Part model, mm, in its own coordinate system. A direction names the side the tool comes from. Round coordinates to 2 decimals unless told otherwise and drop trailing zeros. Order: outer loops, then holes, each group sorted by start corner. A loop starts at its lowest first (then second) coordinate and runs counter-clockwise, first axis right, second up. Notation, with made-up numbers: M -21,86.25 L 0,86.25 A15 cw 0,114.25 Z; hole C 51,45.5 d6. An arc over 180 degrees is marked long. One line per question, with ' | ' between items.
from build123d import *

# Parameters (mm, degrees)
BASE_FLANGE1_DEPTH      = 12.5
CUT_EXTRUDE2_DEPTH      = 64.602279833
CUT_EXTRUDE2_DEPTH_BACK = 64.602279833
SKETCH7_R               = 1.3
SKETCH16_R              = 5
CUT_EXTRUDE5_DEPTH      = 10
SKETCH17_R              = 1.3
CUT_EXTRUDE6_DEPTH      = 10
FILLET3_R               = 2
SKETCH18_W              = 7
SKETCH18_H              = 42.8
CUT_EXTRUDE7_DEPTH      = 71.087445381
FILLET4_R               = 2


# Sheet-metal steps are written as plain solids
with BuildPart() as part:
    # Sketch1 → Base-Flange1 (new, symmetric)
    with BuildSketch(Plane.XY):
        with BuildLine():
            Line((-15, 60), (-15, 3.33))
            ThreePointArc((-15, 3.33), (-14.024665581, 0.975334419), (-11.67, 0))
            Line((-11.67, 0), (11.67, 0))
            ThreePointArc((11.67, 0), (14.024665581, 0.975334419), (15, 3.33))
            Line((15, 3.33), (15, 60))
            Line((15, 60), (17, 60))
            Line((17, 60), (17, 3.33))
            ThreePointArc((17, 3.33), (15.438879144, -0.438879144), (11.67, -2))
            Line((11.67, -2), (-11.67, -2))
            ThreePointArc((-11.67, -2), (-15.438879144, -0.438879144), (-17, 3.33))
            Line((-17, 3.33), (-17, 60))
            Line((-17, 60), (-15, 60))
        make_face()
    extrude(amount=BASE_FLANGE1_DEPTH, both=True)

    # Sketch7 → Cut-Extrude2 (cut, two sides: drawn at the far end of the back side and taken through both)
    with BuildSketch(Plane(origin=(0, 0, 0), x_dir=(0, 0, -1), z_dir=(1, 0, 0)).offset(-CUT_EXTRUDE2_DEPTH_BACK)):
        with Locations((-8.5, 57.4)):
            Circle(SKETCH7_R)
        with Locations((8.5, 57.4)):
            Circle(SKETCH7_R)
    extrude(amount=CUT_EXTRUDE2_DEPTH + CUT_EXTRUDE2_DEPTH_BACK, mode=Mode.SUBTRACT)

    # Sketch16 → Cut-Extrude5 (cut)
    with BuildSketch(Plane.XZ.offset(2)):
        with Locations(Location((0, 0, 0), (0, 0, 270))):
            Circle(SKETCH16_R)
    extrude(amount=-CUT_EXTRUDE5_DEPTH, mode=Mode.SUBTRACT)

    # Sketch17 → Cut-Extrude6 (cut)
    with BuildSketch(Plane(origin=(0, 0, 0), x_dir=(1, 0, 0), z_dir=(0, 1, 0))):
        with Locations(Location((-9, 10, 0), (0, 0, 270))):
            Circle(SKETCH17_R)
        with Locations(Location((9, 10, 0), (0, 0, 270))):
            Circle(SKETCH17_R)
        with Locations(Location((9, -10, 0), (0, 0, 270))):
            Circle(SKETCH17_R)
        with Locations(Location((-9, -10, 0), (0, 0, 270))):
            Circle(SKETCH17_R)
    extrude(amount=-CUT_EXTRUDE6_DEPTH, mode=Mode.SUBTRACT)

    # Fillet3
    fillet3_edges = [part.edges().sort_by_distance(p)[0] for p in [
        (-16, 60, -12.5),
        (16, 60, -12.5),
        (-16, 60, 12.5),
        (16, 60, 12.5),
    ]]
    fillet(fillet3_edges, radius=FILLET3_R)

    # Sketch18 → Cut-Extrude7 (cut, through all)
    with BuildSketch(Plane.ZY.offset(17)):
        with Locations((0, 30)):
            Rectangle(SKETCH18_W, SKETCH18_H)
    extrude(amount=-CUT_EXTRUDE7_DEPTH, mode=Mode.SUBTRACT)

    # Fillet4
    fillet4_edges = [part.edges().sort_by_distance(p)[0] for p in [
        (16, 51.4, 3.5),
        (16, 8.6, 3.5),
        (16, 8.6, -3.5),
        (16, 51.4, -3.5),
        (-16, 51.4, 3.5),
        (-16, 8.6, 3.5),
        (-16, 8.6, -3.5),
        (-16, 51.4, -3.5),
    ]]
    fillet(fillet4_edges, radius=FILLET4_R)


solid = part.part
1) Probe line 1 (X direction, y = 15, z = 10); line 2 (Z direction, x = -15.6, y = 57.4); line 3 (X direction, y = -0.6, z = 10). List the from-to ranges inside material, lowest first. Write a range as [from, to].
The answers:
line 1: x = [-17, -15], [15, 17] | line 2: z = [-12.5, -9.8], [-7.2, 7.2], [9.8, 12.5] | line 3: x = [-15.27, -10.3], [-7.7, 7.7], [10.3, 15.27]
2) Two-plate mould, pull along Y, no slides. Class faces 1 (the face through (16, 8.6, 0)), 2 (the face through (9.39, -0.99, -8.76)), 3 (the face through (-15.99, 50.8, 2.93)), 4 (the face through (-15.4, -0.48, 0.18)): released by +Y, released by -Y, zero draft, split by the parting line, or undercut.
The answers:
face 1: undercut | face 2: zero draft | face 3: undercut | face 4: released by -Y
3) Drop flat-ended pins along their axis: pin 1 (0.6 mm diameter, centred on x = 16, z = 0.5, fed in from -Y); pin 2 (8 mm diameter, centred on x = 9, z = -1, fed in from +Y); pin 3 (3 mm diameter, centred on y = 57.4, z = 8.5, fed in from +X); pin 4 (2 mm diameter, centred on x = 7.5, z = 4.5, fed in from +Y). Give the stop position or say it passes through.
The answers:
pin 1: stops at y = -0.16 | pin 2: stops at y = 0.28 | pin 3: stops at x = 17 | pin 4: stops at y = 0
4) Saw through at B-B (z = 0). List the corners of the cut face in (x, y), plus the area to 3 significant figures.
The answers:
outline: M -17,3.33 A5.33 ccw -11.67,-2 L -5,-2 L -5,0 L -11.67,0 A3.33 cw -15,3.33 L -15,8.6 L -17,8.6 Z; M -17,51.4 L -15,51.4 L -15,60 L -17,60 Z; M 5,-2 L 11.67,-2 A5.33 ccw 17,3.33 L 17,8.6 L 15,8.6 L 15,3.33 A3.33 cw 11.67,0 L 5,0 Z; M 15,51.4 L 17,51.4 L 17,60 L 15,60 Z | area: 109 mm²
5) Saw through at D-D (x = 0). List the corners of the cut face in (y, z), plus the area to 3 significant figures.
The answers:
outline: M -2,-12.5 L 0,-12.5 L 0,-5 L -2,-5 Z; M -2,5 L 0,5 L 0,12.5 L -2,12.5 Z | area: 30.0 mm²
6) Saw through at A-A (y = 23). List the corners of the cut face in (x, z), plus the area to 3 significant figures.
The answers:
outline: M -17,-12.5 L -15,-12.5 L -15,-3.5 L -17,-3.5 Z; M -17,3.5 L -15,3.5 L -15,12.5 L -17,12.5 Z; M 15,-12.5 L 17,-12.5 L 17,-3.5 L 15,-3.5 Z; M 15,3.5 L 17,3.5 L 17,12.5 L 15,12.5 Z | area: 72.0 mm²
7) Which spindle directions (+Z, -Z, +X, -X, +Y, -Y) get a long thin tool onto all of the face, cutting with end or side? Do faces 5 (the face through (14, 0.95, 0.18)), 6 (the face through (9.39, -0.99, 11.24)), 7 (the face through (-15.99, 9.17, 2.9)). Say none if no direction does.
The answers:
face 5: +Z, -Z, +Y | face 6: +Y, -Y | face 7: +X, -X
8) Saw through at C-C (x = -9). List the corners of the cut face in (y, z), plus the area to 3 significant figures.
The answers:
outline: M -2,-12.5 L 0,-12.5 L 0,-11.3 L -2,-11.3 Z; M -2,-8.7 L 0,-8.7 L 0,8.7 L -2,8.7 Z; M -2,11.3 L 0,11.3 L 0,12.5 L -2,12.5 Z | area: 39.6 mm²
